Here's the drawing with two shaded views (mm, measured from the low corner). I have some questions. A direction names the side the tool comes from. Coordinates: 2 decimals unless noted, no trailing zeros. Order: outer loops, then holes, each group sorted by start corner. A loop starts at its lowest first (then second) coordinate and runs counter-clockwise, first axis right, second up. Notation, with made-up numbers: (-33, -5) - (-14, -5) arc R13 cw to (-14, 5) - close; hole circle Ø7 at (-15, -20). An arc over 180 degrees is marked (long way). Answer as CSV lines item,"result". Start each with the question number.
1. I want a section at B-B, the plane z = 7.5. List the corners of the cut face in (x, y) for me, and give its area (3 significant figures).
2. For pin 1 (2.5 mm diameter, centred on x = 7.5, y = 7.5, fed in from -Z); pin 2 (8 mm diameter, centred on x = 5.5, z = 10.5, fed in from +Y), each with a flat end and sliding along its axis, tell me the tip position at first contact or that it passes through.
3. I want a section at C-C, the plane y = 6.75. List the corners of the cut face in (x, z) for me, and give its area (3 significant figures).
4. Thinking about a two-plate mould opening in Y: for the marked faces 3, 4 and 5, which applies, released by +Y, released by -Y, zero draft, split by the parting line, or undercut?
5. I want a section at A-A, the plane x = 7.5. List the corners of the cut face in (y, z) for me, and give its area (3 significant figures).
6. For the marked faces 1 and 2, which set-ups out of +Z, -Z, +X, -X, +Y, -Y let a thin tool reach every point of the face, with its end or its side?
7. I want a section at D-D, the plane x = 4.5. List the corners of the cut face in (y, z) for me, and give its area (3 significant figures).
8. I need wall thicknesses on probe 1 along Y at (x, z) = (7.5, 0.8). Which ranges of the line are inside material? Lowest first, please.
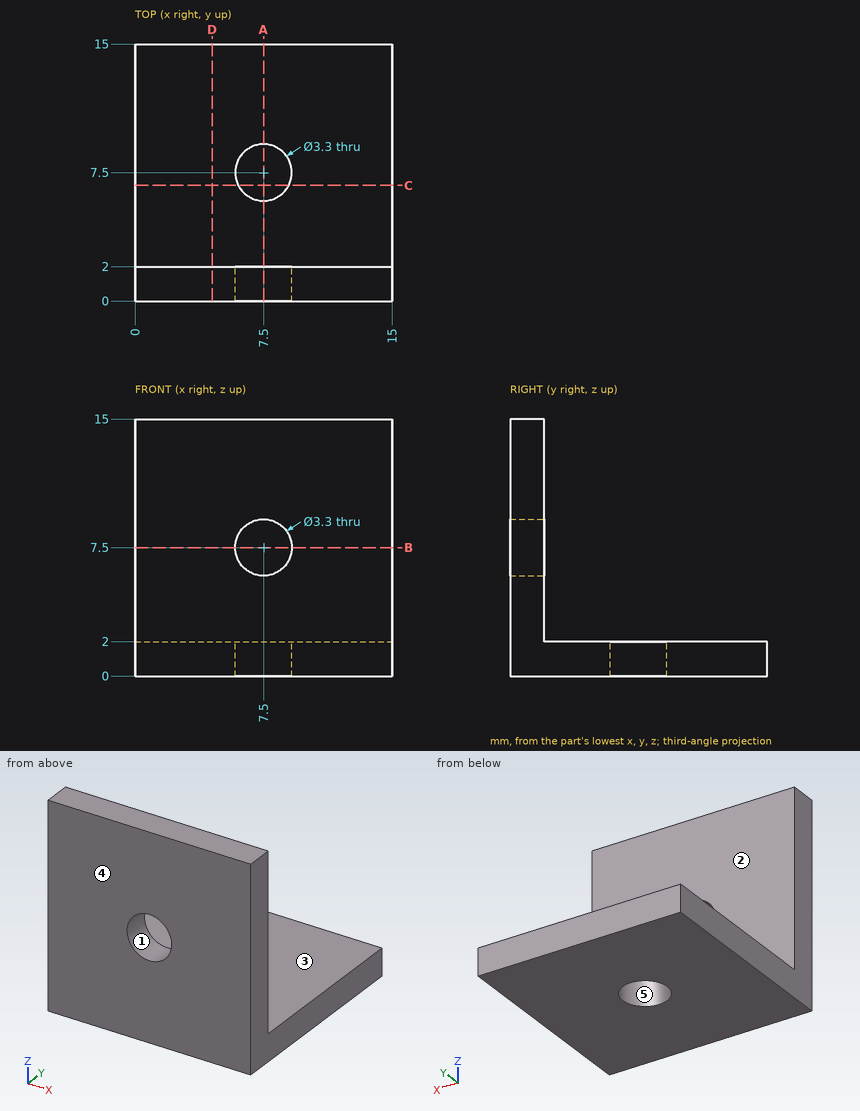
Solved:
1,outline,"(0, 0) - (5.85, 0) - (5.85, 2) - (0, 2) - close; (9.15, 0) - (15, 0) - (15, 2) - (9.15, 2) - close"
1,area,"23.4 mm2"
2,pin 1,"passes through"
2,pin 2,"stops at y = 2"
3,outline,"(0, 0) - (6.03, 0) - (6.03, 2) - (0, 2) - close; (8.97, 0) - (15, 0) - (15, 2) - (8.97, 2) - close"
3,area,"24.1 mm2"
4,face 3,"zero draft"
4,face 4,"released by -Y"
4,face 5,"undercut"
5,outline,"(0, 0) - (5.85, 0) - (5.85, 2) - (2, 2) - (2, 5.85) - (0, 5.85) - close; (0, 9.15) - (2, 9.15) - (2, 15) - (0, 15) - close; (9.15, 0) - (15, 0) - (15, 2) - (9.15, 2) - close"
5,area,"42.8 mm2"
6,face 1,"+Y, -Y"
6,face 2,"+Z, +X, -X, +Y"
7,outline,"(0, 0) - (15, 0) - (15, 2) - (2, 2) - (2, 15) - (0, 15) - close"
7,area,"56.0 mm2"
8,probe 1,"y = 0 to 5.85, 9.15 to 15"
